```python
from build123d import *

# Parameters (mm, degrees)
SKETCH_1_W          = 49
SKETCH_1_H          = 37.5
EXTRUDE_1_DEPTH     = 2
SKETCH_2_R          = 1.5
CUT_EXTRUDE_1_DEPTH = 35.450757188
SKETCH_3_R          = 7
EXTRUDE_2_DEPTH     = 7
SKETCH_4_W          = 13
SKETCH_4_H          = 13.5
EXTRUDE_3_DEPTH     = 6


with BuildPart() as part:
    # Эскиз1 → Бобышка-Вытянуть1 (new body)
    with BuildSketch(Plane.XY):
        with Locations((2.388954836, -2.693851768)):
            Rectangle(SKETCH_1_W, SKETCH_1_H)
    extrude(amount=EXTRUDE_1_DEPTH)

    # Эскиз2 → Вырез-Вытянуть1 (cut, through all)
    with BuildSketch(Plane.XY.offset(2)):
        with Locations((-19.111045164, 13.056148232)):
            Circle(SKETCH_2_R)
        with Locations((23.888954836, 13.056148232)):
            Circle(SKETCH_2_R)
        with Locations((23.888954836, -18.443851768)):
            Circle(SKETCH_2_R)
        with Locations((-19.111045164, -18.443851768)):
            Circle(SKETCH_2_R)
    extrude(amount=-CUT_EXTRUDE_1_DEPTH, mode=Mode.SUBTRACT)

    # Эскиз3 → Бобышка-Вытянуть2 (add)
    with BuildSketch(Plane.XY.offset(2)):
        with Locations((14.888954836, -5.443851768)):
            Circle(SKETCH_3_R)
    extrude(amount=EXTRUDE_2_DEPTH)

    # Эскиз4 → Бобышка-Вытянуть3 (add)
    with BuildSketch(Plane.XY.offset(2)):
        with Locations((-6.411045164, -2.693851768)):
            Rectangle(SKETCH_4_W, SKETCH_4_H)
    extrude(amount=EXTRUDE_3_DEPTH)


solid = part.part
```
Here's how the part is built. I have some questions about the finished solid (model axes, mm). A direction names the side the tool comes from. Coordinates: 2 decimals unless noted, no trailing zeros. Loops run counter-clockwise (first coordinate to the right, second up) from the corner with the lowest first, then second, coordinate; pieces in that order, holes last. Notation, with made-up numbers: (77.5, 84.25) - (128.5, 84.25) arc R37 cw to (128.5, 121.25) - close; hole circle Ø11 at (37, -17). An arc over 180 degrees is marked (long way). Answer as CSV lines item,"result".
Q1. We'd pull the mould along X, two halves only. Please class faces 4 (the face through (-20.61, 13.12, 1.01)), 5 (the face through (-22.111, -3, 1)), 6 (the face through (2, -21.444, 1)), 7 (the face through (-19.436, -19.908, 1.014)): pulls with the +X half, pulls with the -X half, needs draft (parallel to the pull), parting line crosses it, or undercut.
Response:
face 4,"undercut"
face 5,"pulls with the -X half"
face 6,"needs draft"
face 7,"undercut"
Q2. If we section it at D-D, the plane z = 5.75: Write out the boundary of the cut face in (x, y).
Response:
outline,"(-12.91, -9.44) - (0.09, -9.44) - (0.09, 4.06) - (-12.91, 4.06) - close; circle Ø14 at (14.89, -5.44)"
Q3. For pin 1 (3 mm diameter, centred on x = -7, z = 5, fed in from -Y); pin 2 (4 mm diameter, centred on x = 23.89, y = 13.06, fed in from +Z); pin 3 (10.5 mm diameter, centred on x = -6, y = -1.5, fed in from +Z), each with a flat end and sliding along its axis, tell me the tip position at first contact or that it passes through.
Response:
pin 1,"y = -9.44"
pin 2,"z = 2"
pin 3,"z = 8"
Q4. If we section it at B-B, the plane z = 1.5: Write out the boundary of the cut face in (x, y).
Response:
outline,"(-22.11, -21.44) - (26.89, -21.44) - (26.89, 16.06) - (-22.11, 16.06) - close; hole circle Ø3 at (-19.11, -18.44); hole circle Ø3 at (-19.11, 13.06); hole circle Ø3 at (23.89, -18.44); hole circle Ø3 at (23.89, 13.06)"
Q5. If I drill on L1, parallel to Z at x = 14, y = 7; L2, parallel to X at y = -2.5, z = 5; L3, parallel to Y at x = -9, z = 7.25, over which ranges is the centre line in solid material (lowest first)? Write a range as [from, to].
Response:
L1,"[0, 2]"
L2,"[-12.91, 0.09], [8.54, 21.24]"
L3,"[-9.44, 4.06]"
Q6. If we section it at A-A, the plane x = 23.5: Write out the boundary of the cut face in (y, z), and give its area (3 significant figures).
Response:
outline,"(-21.44, 0) - (-19.89, 0) - (-19.89, 2) - (-21.44, 2) - close; (-17, 0) - (11.61, 0) - (11.61, 2) - (-17, 2) - close; (14.5, 0) - (16.06, 0) - (16.06, 2) - (14.5, 2) - close"
area,"63.4 mm2"
Q7. For faces 1 (the face through (7.896, -5.136, 5.451)), 2 (the face through (-7, -3, 8)), 3 (the face through (0.089, -3, 5)), which set-ups out of +Z, -Z, +X, -X, +Y, -Y let a thin tool reach every point of the face, with its end or its side?
Response:
face 1,"+Z"
face 2,"+Z, -X, +Y, -Y"
face 3,"+Z, +Y, -Y"
Q8. If we section it at C-C, the plane y = 3.5: Write out the boundary of the cut face in (x, z), and give its area (3 significant figures).
Response:
outline,"(-22.11, 0) - (26.89, 0) - (26.89, 2) - (0.09, 2) - (0.09, 8) - (-12.91, 8) - (-12.91, 2) - (-22.11, 2) - close"
area,"176 mm2"
